Check sheet for the modelled part. Datum: model origin and axes. Units: mm. A direction names the side the tool comes from. Coordinates: 2 decimals unless noted, no trailing zeros. Order: outer loops, then holes, each group sorted by start corner. A loop starts at its lowest first (then second) coordinate and runs counter-clockwise, first axis right, second up.
1. Thickness scan on line 1 (Z direction, x = -1.75, y = 12); line 2 (X direction, y = 12.25, z = 0.1); line 3 (Y direction, x = -0.15, z = 1.7). Record the ranges inside material, lowest first.
2. Cross-section at D-D (z = 1.05). Enter the section's corners in (x, y).
3. Cross-section at B-B (z = 0.1). Enter the section's corners in (x, y), then the cut area to 3 significant figures.
4. Cross-section at A-A (y = 9.5). Enter the section's corners in (x, z).
5. Set-up check for faces 1 (the flat face through (-1, 11.19, 0)), 2 (the flat face through (-1, 12, 2)), 3 (the flat face through (-1, 12, -2)): record each of +Z, -Z, +X, -X, +Y, -Y from which the full face is reachable in a straight line by a thin tool's end or side.
6. Gauge pin test, flat ends, axial feed: pin 1 Ø1.6 at (x, z) = (-0.5, -1) entering from -Y; pin 2 Ø1 at (x, z) = (-1, 0.5) entering from +Y; pin 3 Ø1.5 at (y, z) = (10.5, -1.5) entering from -X. Record the tip position at first contact, or that the pin passes through.
7. Cross-section at C-C (x = -0.95). Enter the section's corners in (y, z), then the cut area to 3 significant figures.
```python
from build123d import *

# Parameters (mm, degrees)
SKETCH_1_R               = 2.5
EXTRUDE_1_DEPTH          = 23.88
SKETCH_2_R               = 1
EXTRUDE_2_DEPTH          = 1
CUT_EXTRUDE_1_DEPTH      = 5
CUT_EXTRUDE_START        = 18.88
CUT_EXTRUDE_2_DEPTH      = 5
SKETCH_6_R               = 0.25
CUT_EXTRUDE_3_DEPTH      = 0.25
CUT_EXTRUDE_START_2      = 5.25
SKETCH_7_R               = 0.25
CUT_EXTRUDE_4_DEPTH      = 0.25
EXTRUDE_START            = 7
SKETCH_17_R              = 3.5
EXTRUDE_5_DEPTH          = 9.88
CUT_EXTRUDE_6_DEPTH      = 26.937509518
CUT_EXTRUDE_6_DEPTH_BACK = 26.937509518
SKETCH_20_OUTSIDE_W      = 20.616
SKETCH_20_OUTSIDE_H      = 31.496
SKETCH_20_OUTSIDE_W_2    = 7
SKETCH_20_OUTSIDE_H_2    = 9.88
CUT_EXTRUDE_7_DEPTH      = 18.590747568
CUT_EXTRUDE_7_DEPTH_BACK = 18.590747568
SKETCH_22_W              = 5.5
SKETCH_22_H              = 9.88
EXTRUDE_START_2          = -2
SKETCH_24_W              = 4
SKETCH_24_H              = 1.5
EXTRUDE_6_DEPTH          = 2


with BuildPart() as part:
    # 草图1 → 凸台-拉伸1 (new body)
    with BuildSketch(Plane(origin=(0, 0, 0), x_dir=(1, 0, 0), z_dir=(0, 1, 0))):
        with Locations(Location((0, 0, 0), (0, 0, 90))):
            Circle(SKETCH_1_R)
    extrude(amount=EXTRUDE_1_DEPTH)

    # 草图2 → 凸台-拉伸2 (add)
    with BuildSketch(Plane(origin=(0, 0, 0), x_dir=(1, 0, 0), z_dir=(0, 1, 0))):
        with BuildLine():
            Line((0.166666667, 2.494438258), (7.633333333, 1.995550606))
            ThreePointArc((7.633333333, 1.995550606), (9.5, 0), (7.633333333, -1.995550606))
            Line((7.633333333, -1.995550606), (0.166666667, -2.494438258))
            ThreePointArc((0.166666667, -2.494438258), (-2.5, 0), (0.166666667, 2.494438258))
        make_face()
        with Locations(Location((7.5, 0, 0), (0, 0, 270))):
            Circle(SKETCH_2_R, mode=Mode.SUBTRACT)
    extrude(amount=EXTRUDE_2_DEPTH)

    # 草图3 → 切除-拉伸1 (cut)
    with BuildSketch(Plane(origin=(0, 0, 0), x_dir=(1, 0, 0), z_dir=(0, 1, 0))):
        with BuildLine():
            Line((-1.854049622, -0.75), (-0.75, -0.75))
            Line((-0.75, -0.75), (-0.75, -1.854049622))
            ThreePointArc((-0.75, -1.854049622), (0, -2), (0.75, -1.854049622))
            Line((0.75, -1.854049622), (0.75, -0.75))
            Line((0.75, -0.75), (1.854049622, -0.75))
            ThreePointArc((1.854049622, -0.75), (2, 0), (1.854049622, 0.75))
            Line((1.854049622, 0.75), (0.75, 0.75))
            Line((0.75, 0.75), (0.75, 1.854049622))
            ThreePointArc((0.75, 1.854049622), (0, 2), (-0.75, 1.854049622))
            Line((-0.75, 1.854049622), (-0.75, 0.75))
            Line((-0.75, 0.75), (-1.854049622, 0.75))
            ThreePointArc((-1.854049622, 0.75), (-2, 0), (-1.854049622, -0.75))
        make_face()
    extrude(amount=CUT_EXTRUDE_1_DEPTH, mode=Mode.SUBTRACT)

    # 草图5 → 切除-拉伸2 (cut)
    with BuildSketch(Plane(origin=(0, 0, 0), x_dir=(1, 0, 0), z_dir=(0, 1, 0)).offset(CUT_EXTRUDE_START)):
        with BuildLine():
            Line((1.854049622, 0.75), (0.75, 0.75))
            Line((0.75, 0.75), (0.75, 1.854049622))
            ThreePointArc((0.75, 1.854049622), (0, 2), (-0.75, 1.854049622))
            Line((-0.75, 1.854049622), (-0.75, 0.75))
            Line((-0.75, 0.75), (-1.854049622, 0.75))
            ThreePointArc((-1.854049622, 0.75), (-2, 0), (-1.854049622, -0.75))
            Line((-1.854049622, -0.75), (-0.75, -0.75))
            Line((-0.75, -0.75), (-0.75, -1.854049622))
            ThreePointArc((-0.75, -1.854049622), (0, -2), (0.75, -1.854049622))
            Line((0.75, -1.854049622), (0.75, -0.75))
            Line((0.75, -0.75), (1.854049622, -0.75))
            ThreePointArc((1.854049622, -0.75), (2, 0), (1.854049622, 0.75))
        make_face()
    extrude(amount=CUT_EXTRUDE_2_DEPTH, mode=Mode.SUBTRACT)

    # 草图6 → 切除-拉伸3 (cut)
    with BuildSketch(Plane(origin=(0, 0, 0), x_dir=(1, 0, 0), z_dir=(0, 1, 0)).offset(CUT_EXTRUDE_START)):
        with Locations(Location((0.75, 0, 0), (0, 0, 270))):
            Circle(SKETCH_6_R)
    extrude(amount=-CUT_EXTRUDE_3_DEPTH, mode=Mode.SUBTRACT)

    # 草图7 → 切除-拉伸4 (cut)
    with BuildSketch(Plane(origin=(0, 0, 0), x_dir=(1, 0, 0), z_dir=(0, 1, 0)).offset(CUT_EXTRUDE_START_2)):
        with Locations(Location((0.75, 0, 0), (0, 0, 270))):
            Circle(SKETCH_7_R)
    extrude(amount=-CUT_EXTRUDE_4_DEPTH, mode=Mode.SUBTRACT)

    # 草图17 → 凸台-拉伸5 (add)
    with BuildSketch(Plane(origin=(0, 0, 0), x_dir=(1, 0, 0), z_dir=(0, 1, 0)).offset(EXTRUDE_START)):
        with Locations(Location((0, 0, 0), (0, 0, 270))):
            Circle(SKETCH_17_R)
    extrude(amount=EXTRUDE_5_DEPTH)

    # 草图20 outside → 切除-拉伸6 (cut, two sides: drawn at the far end of the back side and taken through both)
    with BuildSketch(Plane.XY.offset(-CUT_EXTRUDE_6_DEPTH_BACK)):
        with Locations((3, 11.94)):
            Rectangle(SKETCH_20_OUTSIDE_W, SKETCH_20_OUTSIDE_H)
        with Locations((0, 11.94)):
            Rectangle(SKETCH_20_OUTSIDE_W_2, SKETCH_20_OUTSIDE_H_2, mode=Mode.SUBTRACT)
    extrude(amount=CUT_EXTRUDE_6_DEPTH + CUT_EXTRUDE_6_DEPTH_BACK, mode=Mode.SUBTRACT)

    # 草图22 → 切除-拉伸7 (cut, two sides: drawn at the far end of the back side and taken through both)
    with BuildSketch(Plane.XY.offset(-CUT_EXTRUDE_7_DEPTH_BACK)):
        with Locations((0.75, 11.94)):
            Rectangle(SKETCH_22_W, SKETCH_22_H)
    extrude(amount=CUT_EXTRUDE_7_DEPTH + CUT_EXTRUDE_7_DEPTH_BACK, mode=Mode.SUBTRACT)

    # 草图24 → 凸台-拉伸6 (add)
    with BuildSketch(Plane(origin=(0, 0, 0), x_dir=(0, 0, -1), z_dir=(1, 0, 0)).offset(EXTRUDE_START_2)):
        with Locations((0, 11.94)):
            Rectangle(SKETCH_24_W, SKETCH_24_H)
    extrude(amount=EXTRUDE_6_DEPTH)


solid = part.part
```
Data:
1. line 1: z = -2 to 2
1. line 2: x = -3.5 to 0
1. line 3: y = 11.19 to 12.69
2. outline: (-3.34, 7) - (-2, 7) - (-2, 11.19) - (0, 11.19) - (0, 12.69) - (-2, 12.69) - (-2, 16.88) - (-3.34, 16.88) - close
3. outline: (-3.5, 7) - (-2, 7) - (-2, 11.19) - (0, 11.19) - (0, 12.69) - (-2, 12.69) - (-2, 16.88) - (-3.5, 16.88) - close
3. area: 17.8 mm2
4. outline: (-2, -2.87) - (-2, 2.87) arc R3.5 ccw to start
5. face 1: +Z, -Z, +X, -Y
5. face 2: +Z, +X, +Y, -Y
5. face 3: -Z, +X, +Y, -Y
6. pin 1: stops at y = 11.19
6. pin 2: stops at y = 12.69
6. pin 3: stops at x = -3.42
7. outline: (11.19, -2) - (12.69, -2) - (12.69, 2) - (11.19, 2) - close
7. area: 6.00 mm2
